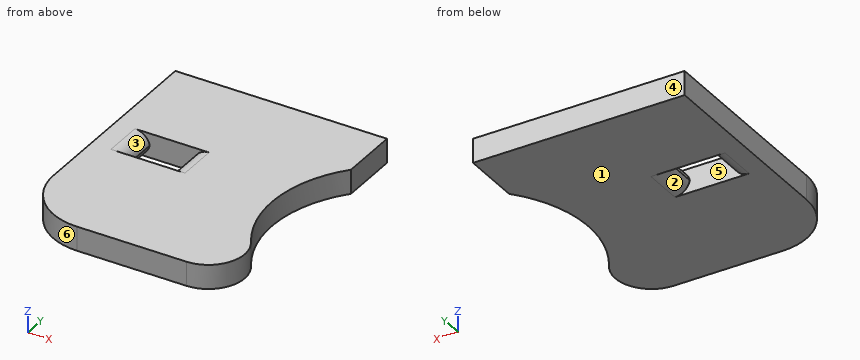
```python
from build123d import *

# Parameters (mm, degrees)
BOSS_EXTRU_1_DEPTH      = 4
ESQUISSE2_W             = 7.25
ESQUISSE2_H             = 6.5
ENL_V_MAT_EXTRU_1_DEPTH = 96.785571069
CONG_1_R                = 2.5
CUT_EXTRUDE1_REACH      = 97.786


with BuildPart() as part:
    # Esquisse1 → Boss.-Extru.1 (new body)
    with BuildSketch(Plane.XY):
        with BuildLine():
            Line((-34.444097209, -52.025), (-34.444097209, -52.525))
            Line((-34.444097209, -52.525), (-70, -52.525))
            ThreePointArc((-70, -52.525), (-77.071067812, -49.596067812), (-80, -42.525))
            Line((-80, -42.525), (-80, -9.525))
            Line((-80, -9.525), (-45, -9.525))
            Line((-45, -9.525), (-45, -19.296243445))
            ThreePointArc((-45, -19.296243445), (-49.034471505, -38.664128156), (-34.444097209, -52.025))
        make_face()
    extrude(amount=BOSS_EXTRU_1_DEPTH)

    # Esquisse2 → Enlèv. mat.-Extru.1 (cut, through all)
    with BuildSketch(Plane(origin=(0, 0, 0), x_dir=(-1, 0, 0), z_dir=(0, 0, -1))):
        with Locations((70.625, -29.025)):
            Rectangle(ESQUISSE2_W, ESQUISSE2_H)
    extrude(amount=-ENL_V_MAT_EXTRU_1_DEPTH, mode=Mode.SUBTRACT)

    # Congé1
    # the kernel refuses this fillet: 2.5 mm, written as the material it takes off along each edge
    with BuildSketch(Plane(origin=(-74.25, -25.775, 4), x_dir=(-1, 0, 0), z_dir=(0, -1, 0)), Plane(origin=(-67, -32.275, 4), x_dir=(1, 0, 0), z_dir=(0, 1, 0))) as cong_1_piece_1:
        with BuildLine():
            CenterArc((CONG_1_R, CONG_1_R), CONG_1_R, 180, 90)
            Line((0, CONG_1_R), (0, 0))
            Line((0, 0), (CONG_1_R, 0))
        make_face()
    extrude(amount=6.5, mode=Mode.SUBTRACT)
    with BuildSketch(Plane(origin=(-74.25, -25.775, 0), x_dir=(-1, 0, 0), z_dir=(0, -1, 0)), Plane(origin=(-67, -32.275, 0), x_dir=(1, 0, 0), z_dir=(0, 1, 0))) as cong_1_piece_2:
        with BuildLine():
            CenterArc((CONG_1_R, -CONG_1_R), CONG_1_R, 90, 90)
            Line((0, -CONG_1_R), (0, 0))
            Line((0, 0), (CONG_1_R, 0))
        make_face()
    extrude(amount=6.5, mode=Mode.SUBTRACT)

    # Sketch1 → Cut-Extrude1 (cut, up to next)
    with BuildSketch(Plane(origin=(0, 0, 0), x_dir=(-1, 0, 0), z_dir=(0, 0, -1)), mode=Mode.PRIVATE) as cut_extrude1_sk1:
        with BuildLine():
            Line((51.9089023, -52.525), (34.444097209, -52.525))
            Line((34.444097209, -52.525), (34.444097209, -52.025))
            Line((34.444097209, -52.025), (46.853001769, -43.294230769))
            ThreePointArc((46.853001769, -43.294230769), (46.646554184, -49.407306768), (51.9089023, -52.525))
        make_face()
    cut_extrude1_tool1 = extrude(cut_extrude1_sk1.sketch, amount=-CUT_EXTRUDE1_REACH, mode=Mode.PRIVATE) & part.part
    add(cut_extrude1_tool1.solids().sort_by_distance((-42.611695, -49.79665, 0))[0], mode=Mode.SUBTRACT)


solid = part.part
```
Could you check a few things on this model? Use its own coordinates, in mm. Face numbers are marked on the shaded views. A direction names the side the tool comes from. Coordinates: 2 decimals unless noted, no trailing zeros. Write each loop counter-clockwise with the first axis right and the second up, starting at its lowest first coordinate (ties: lowest second). Pieces come first, ordered by that corner, then holes. Notation, with made-up numbers: (77, 55) -> (105, 55) arc R18 cw to (105, 86) -> close; hole circle Ø5 at (56, 85.5). An arc over 180 degrees is marked (long way). Return JSON: item names as keys, results as strings.
(1) I need wall thicknesses on L1, parallel to Y at x = -69, z = 3.2 (3 decimals); L2, parallel to Y at x = -73, z = 3.1 (3 decimals); L3, parallel to X at y = -30, z = 3.65. Which ranges of each line are inside material? Lowest first, please.
Numbers:
{"L1": "y = -52.525 to -32.275, -25.775 to -9.525", "L2": "y = -52.064 to -32.275, -25.775 to -9.525", "L3": "x = -80 to -75.47, -65.78 to -49.84"}
(2) Imagine slicing it at A-A, the plane x = -69.5. Please give me the cut outline in (y, z) (3 decimals), then the cut area to 3 significant figures.
Numbers:
{"outline": "(-52.525, 0) -> (-32.275, 0) -> (-32.275, 4) -> (-52.525, 4) -> close; (-25.775, 0) -> (-9.525, 0) -> (-9.525, 4) -> (-25.775, 4) -> close", "area": "146 mm2"}
(3) Which directions (+Z, -Z, +X, -X, +Y, -Y) give clear straight access to the entire face, cutting with the end or side of a thin tool? Please do the marked faces 1 and 2.
Numbers:
{"face 1": "-Z, +X, -X, +Y, -Y", "face 2": "-Z"}
(4) Imagine slicing it at D-D, the plane x = -66. Please give me the cut outline in (y, z) (3 decimals).
Numbers:
{"outline": "(-52.525, 0) -> (-32.275, 0) -> (-32.275, 0.5) -> (-25.775, 0.5) -> (-25.775, 0) -> (-9.525, 0) -> (-9.525, 4) -> (-25.775, 4) -> (-25.775, 3.5) -> (-32.275, 3.5) -> (-32.275, 4) -> (-52.525, 4) -> close"}
(5) Imagine slicing it at C-C, the plane z = 1.35. Please give me the cut outline in (x, y) (3 decimals), then the cut area to 3 significant figures.
Numbers:
{"outline": "(-80, -42.525) arc R10 ccw to (-70, -52.525) -> (-51.909, -52.525) arc R6 ccw to (-46.853, -43.294) arc R20 cw to (-45, -19.296) -> (-45, -9.525) -> (-80, -9.525) -> close; hole (-74.53, -32.275) -> (-66.72, -32.275) -> (-66.72, -25.775) -> (-74.53, -25.775) -> close", "area": "1,330 mm2"}
(6) I'm going to push flat-ended pins straight in: pin 1 (1 mm diameter, centred on y = -20, z = 3.5, fed in from +X); pin 2 (6 mm diameter, centred on x = -57.5, y = -19.5, fed in from -Z); pin 3 (1.5 mm diameter, centred on x = -48.5, y = -31, fed in from -Z). Where does each tip first touch, or does it pass through?
Numbers:
{"pin 1": "stops at x = -45.18", "pin 2": "stops at z = 0", "pin 3": "passes through"}
(7) Imagine slicing it at B-B, the plane y = -28.5. Please give me the cut outline in (x, z).
Numbers:
{"outline": "(-80, 0) -> (-76.75, 0) arc R2.5 ccw to (-74.3, 2) arc R2.5 ccw to (-76.75, 4) -> (-80, 4) -> close; (-66.95, 2) arc R2.5 ccw to (-64.5, 0) -> (-49.59, 0) -> (-49.59, 4) -> (-64.5, 4) arc R2.5 ccw to start"}
(8) We'd pull the mould along X, two halves only. Please class the marked faces 3, 4, 5 and 6: +X half, -X half, draft (parallel to the pull), parting line (faces both ways), or undercut.
Numbers:
{"face 3": "undercut", "face 4": "draft", "face 5": "undercut", "face 6": "-X half"}
